```python
from build123d import *

# Parameters (mm, degrees)
SKETCH1_R               = 1
BOSS_EXTRUDE1_DEPTH     = 12
SKETCH2_R               = 3.3
CUT_EXTRUDE1_DEPTH      = 4.5
SKETCH3_R               = 3.3
CUT_EXTRUDE2_DEPTH      = 2.5
CUT_EXTRUDE2_DEPTH_BACK = 2.5
FILLET1_R               = 0.5
FILLET2_R               = 1


with BuildPart() as part:
    # Sketch1 → Boss-Extrude1 (new body)
    with BuildSketch(Plane.XY):
        with BuildLine():
            Line((-2.048815827, 41.884151299), (-2.048815827, 23.656682303))
            ThreePointArc((-2.048815827, 23.656682303), (1.66754925, 20.218418642), (3.205412143, 25.042110601))
            add(Edge.make_bspline(
                [(1.896008332, 44.529660516), (1.616069448, 41.758878479), (-0.936917255, 33.955197005), (6.844694938, 29.417505011), (3.205412143, 25.042110601)],
                knots=[0, 0, 0, 0, 0.461184527, 1, 1, 1, 1], degree=3))
            ThreePointArc((1.896008332, 44.529660516), (-2.768270934, 47.220856283), (-2.048815827, 41.884151299))
        make_face()
        with Locations((-1.097343641, 44.729270045)):
            Circle(SKETCH1_R, mode=Mode.SUBTRACT)
        with Locations((0.902656359, 23.119270045)):
            Circle(SKETCH1_R, mode=Mode.SUBTRACT)
        with BuildLine():
            Line((-0.031319306, 41.884151299), (-0.548815827, 41.884151299))
            Line((-0.548815827, 41.884151299), (-0.548815827, 25.744765902))
            ThreePointArc((-0.548815827, 25.744765902), (0.697826573, 26.112269337), (1.982912704, 25.918028026))
            add(Edge.make_bspline(
                [(-0.031319306, 41.884151299), (-0.050798368, 41.769911378), (-0.110231132, 41.41757497), (-0.243210983, 40.585051968), (-0.402027872, 39.353261852), (-0.479087992, 37.828213551), (-0.375856847, 36.275358456), (0.009969142, 34.681069755), (0.941317901, 32.770668216), (2.035404053, 31.246938586), (2.80471042, 29.909471533), (3.128629571, 29.030940173), (3.19641087, 28.267404516), (3.032335606, 27.550309668), (2.666289508, 26.829120101), (2.334869511, 26.350170873), (2.106769915, 26.067173099), (2.026097439, 25.969974031), (1.996829195, 25.934759382), (1.982912704, 25.918028026)],
                knots=[0.149200089, 0.149200089, 0.149200089, 0.149200089, 0.165683382, 0.19960026, 0.265533433, 0.331466606, 0.397399778, 0.463332951, 0.529266124, 0.661132469, 0.727065642, 0.792998815, 0.858931987, 0.92486516, 0.957831746, 0.990798333, 0.999039979, 1.001358499, 1.00341891, 1.00341891, 1.00341891, 1.00341891], degree=3))
        make_face(mode=Mode.SUBTRACT)
    extrude(amount=BOSS_EXTRUDE1_DEPTH)

    # Sketch2 → Cut-Extrude1 (cut)
    with BuildSketch(Plane.XY.offset(12)):
        with Locations((-1.097343641, 44.729270045)):
            Circle(SKETCH2_R)
    cut_extrude1 = extrude(amount=-CUT_EXTRUDE1_DEPTH, mode=Mode.SUBTRACT)

    # Mirror1: Cut-Extrude1 across plane
    add(cut_extrude1.mirror(Plane.XY.offset(6)), mode=Mode.SUBTRACT)

    # Sketch3 → Cut-Extrude2 (cut, two sides)
    with BuildSketch(Plane.XY.offset(6)) as cut_extrude2_sk:
        with Locations((0.902656359, 23.119270045)):
            Circle(SKETCH3_R)
    extrude(amount=CUT_EXTRUDE2_DEPTH, mode=Mode.SUBTRACT)
    extrude(cut_extrude2_sk.sketch, amount=-CUT_EXTRUDE2_DEPTH_BACK, mode=Mode.SUBTRACT)

    # Fillet1
    fillet1_edges = [part.edges().sort_by_distance(p)[0] for p in [
        (1.670824854, 42.932817101, 9.75),
        (-2.048815827, 41.569412346, 9.75),
        (1.670824854, 42.932817101, 2.25),
        (-2.048815827, 41.569412346, 2.25),
    ]]
    fillet(fillet1_edges, radius=FILLET1_R)

    # Fillet2
    fillet2_edges = [part.edges().sort_by_distance(p)[0] for p in [
        (-2.048815827, 41.884151299, 6),
    ]]
    fillet(fillet2_edges, radius=FILLET2_R)


solid = part.part
```
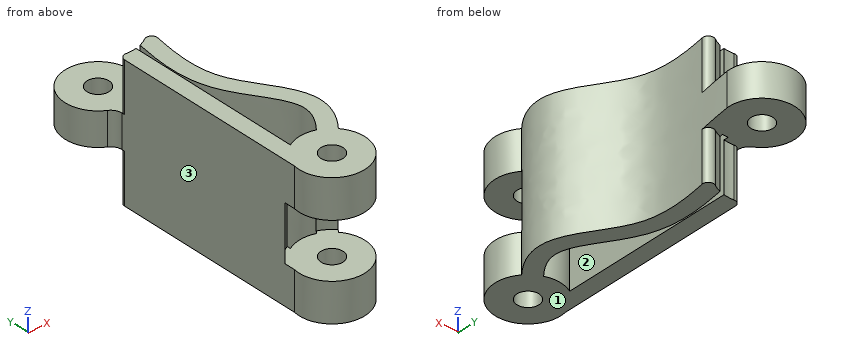
Model file for the job. Use its own axes, mm. Face numbers are marked on the shaded views. Coordinates: 2 decimals unless noted, no trailing zeros. Loops run counter-clockwise (first coordinate to the right, second up) from the corner with the lowest first, then second, coordinate; pieces in that order, holes last. Notation, with made-up numbers: (-30.5, 72) -> (-18.5, 72) arc R27 ccw to (-18.5, 93) -> close; hole circle Ø2 at (-12.75, 13). An arc over 180 degrees is marked (long way). Answer as a JSON object with one key per item and string values.
Q1. Cut at A-A (x = -1). List the corners of the cut face in (y, z), and give its area (3 significant figures).
Report:
{"outline": "(20.8, 0) -> (41.43, 0) -> (41.43, 4.5) -> (43.73, 4.5) -> (43.73, 7.5) -> (41.43, 7.5) -> (41.43, 12) -> (20.8, 12) -> (20.8, 8.5) -> (25.82, 8.5) -> (25.82, 3.5) -> (20.8, 3.5) -> close; (45.72, 4.5) -> (47.73, 4.5) -> (47.73, 7.5) -> (45.72, 7.5) -> close", "area": "235 mm2"}
Q2. Probe probe 1 along Z at (x, y) = (2.5, 25.75); probe 2 along Y at (x, z) = (2.75, 5); probe 3 along X at (y, z) = (27, 6.75). List the from-to ranges inside material, lowest first.
Report:
{"probe 1": "z = 0 to 3.5, 8.5 to 12", "probe 2": "y = 25.85 to 27.01, 29.96 to 32.84", "probe 3": "x = -2.05 to -0.55, 2.75 to 4.39"}
Q3. Flat gauge pins, fed straight in: P1, Ø2, axis at y = 29.5, z = 10, coming from the +X side; P2, Ø2, axis at y = 33.5, z = 10, coming from the +X side; P3, Ø3, axis at y = 31, z = 10.5, coming from the -X side; P4, Ø2, axis at x = 0.5, z = 2, coming from the +Y side. Where does each tip first touch, or does it go through?
Report:
{"P1": "stops at x = 4.66", "P2": "stops at x = 2.97", "P3": "stops at x = -2.05", "P4": "stops at y = 42.01"}
Q4. Pull direction X, two halves, no side cores. Call the marked faces 1, 2 and 3: released by +X, released by -X, zero draft, split by the parting line, or undercut.
Report:
{"face 1": "zero draft", "face 2": "undercut", "face 3": "released by -X"}
